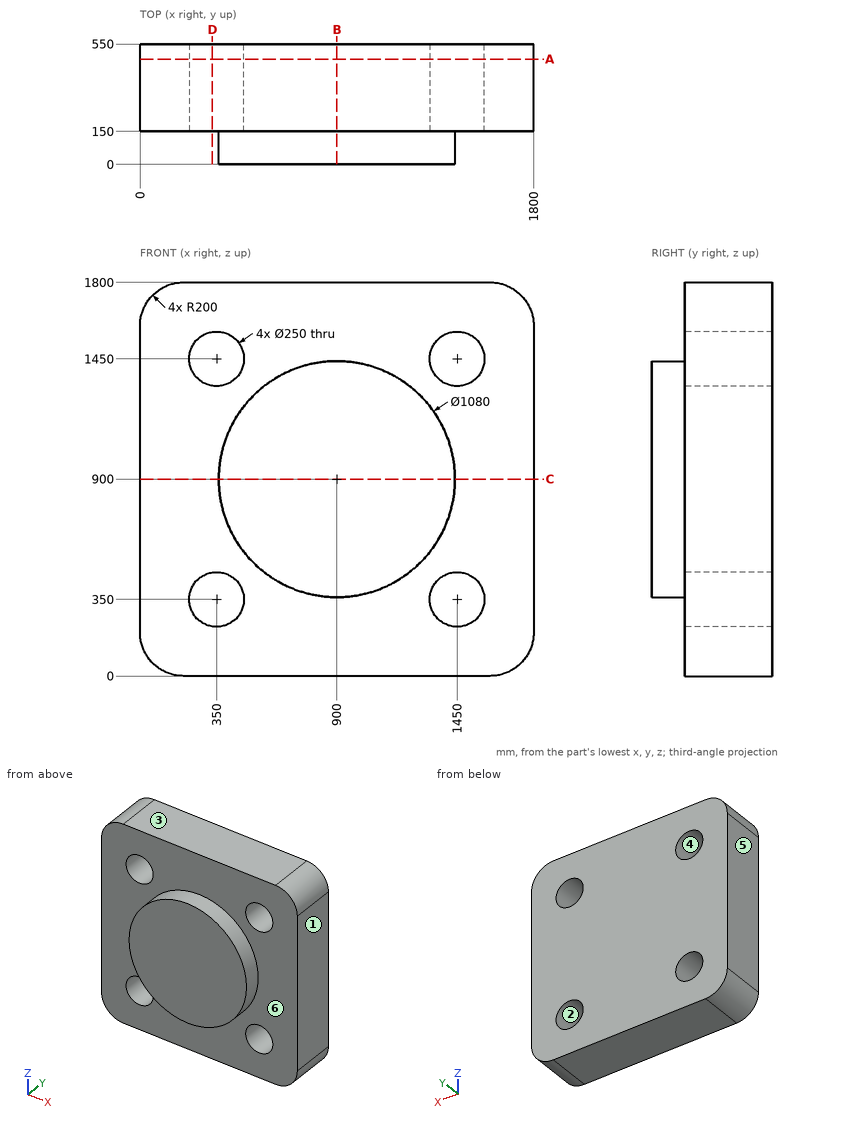
The drawing under review shows one solid part. Ordinate dimensions are in mm from its lowest x, y, z. A direction names the side the tool comes from. Coordinates: 2 decimals unless noted, no trailing zeros. Loops run counter-clockwise (first coordinate to the right, second up) from the corner with the lowest first, then second, coordinate; pieces in that order, holes last. Notation, with made-up numbers: (-25, 83.5) -> (6, 83.5) arc R10 cw to (6, 97.5) -> close; hole circle Ø11 at (-11.75, 56). An arc over 180 degrees is marked (long way). Answer as a JSON object with one key per item and string values.
Q1. Take a section at D-D on x = 331. Give the boundary of the cut face in (y, z), plus the area to 3 significant figures.
Answer block:
{"outline": "(150, 0) -> (550, 0) -> (550, 226.45) -> (150, 226.45) -> close; (150, 473.55) -> (550, 473.55) -> (550, 1326.45) -> (150, 1326.45) -> close; (150, 1573.55) -> (550, 1573.55) -> (550, 1800) -> (150, 1800) -> close", "area": "522,000 mm^2"}
Q2. Tool access review of the marked faces 5 and 6: name each direction out of +Z, -Z, +X, -X, +Y, -Y from which nothing blocks a thin tool from reaching the whole face with its end or side.
Answer block:
{"face 5": "+Z, -Z, -X, +Y, -Y", "face 6": "-Y"}
Q3. To check wall thickness, follow L1, parallel to Z at x = 350, y = 269; L2, parallel to Z at x = 262.5, y = 285. State the ranges of each line that lie inside material, in increasing order.
Answer block:
{"L1": "z = 0 to 225, 475 to 1325, 1575 to 1800", "L2": "z = 0 to 260.73, 439.27 to 1360.73, 1539.27 to 1800"}
Q4. Clearance check with flat-ended pins moving along their axes: pin 1 Ø4 at (x, z) = (1326.5, 434.5) entering from -Y; pin 2 Ø6 at (y, z) = (83.5, 1328.5) entering from -X. State where each tip first meets the part, or that it passes through.
Answer block:
{"pin 1": "stops at y = 150", "pin 2": "stops at x = 567.51"}
Q5. Take a section at A-A on y = 481. Give the boundary of the cut face in (x, z), plus the area to 3 significant figures.
Answer block:
{"outline": "(0, 200) arc R200 ccw to (200, 0) -> (1600, 0) arc R200 ccw to (1800, 200) -> (1800, 1600) arc R200 ccw to (1600, 1800) -> (200, 1800) arc R200 ccw to (0, 1600) -> close; hole circle Ø250 at (350, 350); hole circle Ø250 at (350, 1450); hole circle Ø250 at (1450, 350); hole circle Ø250 at (1450, 1450)", "area": "3,010,000 mm^2"}
Q6. Take a section at B-B on x = 900. Give the boundary of the cut face in (y, z).
Answer block:
{"outline": "(0, 360) -> (150, 360) -> (150, 0) -> (550, 0) -> (550, 1800) -> (150, 1800) -> (150, 1440) -> (0, 1440) -> close"}
Q7. The part is to be moulded in two halves that separate along Z. For the marked faces 1, 2, 3 and 4, say which applies: +Z half, -Z half, draft (parallel to the pull), parting line (faces both ways), or undercut.
Answer block:
{"face 1": "draft", "face 2": "undercut", "face 3": "+Z half", "face 4": "undercut"}
Q8. Take a section at C-C on z = 900. Give the boundary of the cut face in (x, y).
Answer block:
{"outline": "(0, 150) -> (360, 150) -> (360, 0) -> (1440, 0) -> (1440, 150) -> (1800, 150) -> (1800, 550) -> (0, 550) -> close"}
